from build123d import *

# Parameters (mm, degrees)
F1_DEPTH = 19.05
F2_DEPTH = 19.05
F3_DEPTH = 25.4


with BuildPart() as f1:
    # F0 (on Top) → F1 (new body)
    with BuildSketch(Plane.XY):
        with BuildLine():
            ThreePointArc((10.16, 0), (-4.399409, 9.1581), (-6.35, -7.931147))
            ThreePointArc((-6.35, -7.931147), (0, -10.16), (6.35, -7.931147))
            ThreePointArc((6.35, -7.931147), (9.1581, -4.399409), (10.16, 0))
        make_face()
    extrude(amount=F1_DEPTH)

    # F0 (on Top) → F2 (join)
    with BuildSketch(Plane.XY):
        with BuildLine():
            Line((-6.35, -7.931147), (-6.35, -24.593444))
            ThreePointArc((-6.35, -24.593444), (0, -25.4), (6.35, -24.593444))
            Line((6.35, -24.593444), (6.35, -7.931147))
            ThreePointArc((6.35, -7.931147), (0, -10.16), (-6.35, -7.931147))
        make_face()
    extrude(amount=F2_DEPTH)

    # F0 (on Top) → F3 (join)
    with BuildSketch(Plane.XY):
        with BuildLine():
            ThreePointArc((6.35, -24.593444), (20.080463, -15.55426), (25.4, 0))
            ThreePointArc((25.4, 0), (-15.55426, 20.080463), (-6.35, -24.593444))
            Line((-6.35, -24.593444), (-6.35, -7.931147))
            ThreePointArc((-6.35, -7.931147), (-4.399409, 9.1581), (10.16, 0))
            ThreePointArc((10.16, 0), (9.1581, -4.399409), (6.35, -7.931147))
            Line((6.35, -7.931147), (6.35, -24.593444))
        make_face()
    extrude(amount=F3_DEPTH)


solid = f1.part
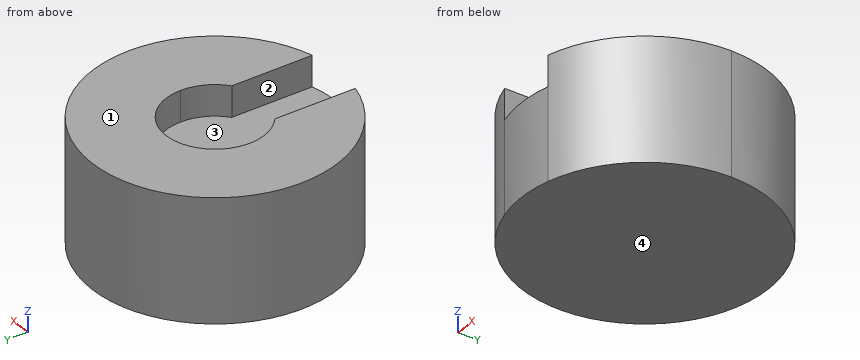
Work out the finished part from the listing and answer in its coordinate system (mm). Face numbers are marked on the shaded views. A direction names the side the tool comes from. Round coordinates to 2 decimals unless told otherwise and drop trailing zeros. Order: outer loops, then holes, each group sorted by start corner. A loop starts at its lowest first (then second) coordinate and runs counter-clockwise, first axis right, second up. Notation, with made-up numbers: M 3,62.5 L 29,62.5 A24 cw 29,83.5 Z; hole C 71,74.25 d6. An arc over 180 degrees is marked long. Put each result on its own line as item: value. Start each with the question number.
Q1. Section B-B, the plane y = -1.5 is taken. Write down the section's boundary in (x, z), and give its area (3 significant figures).
Q2. Straight lines are drawn through the part: L1, parallel to X at y = 0, z = 22.75; L2, parallel to Y at x = 0, z = 23.25; L3, parallel to X at y = 0.5, z = 16.5. For each, find the intervals that lie inside material, in ascending order. Write a range as [from, to].
Q3. Section D-D, the plane y = 8.5 is taken. Write down the section's boundary in (x, z), and give its area (3 significant figures).
Q4. Section C-C, the plane z = 7.75 is taken. Write down the section's boundary in (x, y), and give its area (3 significant figures).
Q5. A tool of negligible diameter and unlimited length cuts with its end or side. For the marked faces 3 and 4, from which of +Z, -Z, +X, -X, +Y, -Y can it reach the whole face along a straight path? Write none if from no direction.
Q6. Section A-A, the plane x = 0 is taken. Write down the section's boundary in (y, z), and give its area (3 significant figures).
Q7. Flat-ended cylindrical pins translate along their axes: pin 1 (10 mm diameter, centred on y = 11, z = 6.5, fed in from -X); pin 2 (4 mm diameter, centred on y = 5, z = 21.5, fed in from +X); pin 3 (5 mm diameter, centred on x = -16, z = 5.5, fed in from -Y). Find the tip coordinate at first contact, or state that the pin passes through.
Q8. For a pull along X with two mould halves and no side action, classify the marked faces 1 and 2 as pulls with the +X half, pulls with the -X half, needs draft (parallel to the pull), parting line crosses it, or undercut.
Findings below:
1. outline: M -25.36,0 L 25.36,0 L 25.36,25.4 L 10.05,25.4 L 10.05,19.05 L -10.05,19.05 L -10.05,25.4 L -25.36,25.4 Z
1. area: 1,160 mm^2
2. L1: x = [-25.4, -10.16], [10.16, 25.4]
2. L2: y = [10.16, 25.4]
2. L3: x = [-25.4, 25.4]
3. outline: M -23.94,0 L 23.94,0 L 23.94,25.4 L 5.57,25.4 L 5.57,19.05 L -5.57,19.05 L -5.57,25.4 L -23.94,25.4 Z
3. area: 1,150 mm^2
4. outline: M -6.35,-24.59 A25.4 ccw 6.35,-24.59 A25.4 ccw long Z
4. area: 2,030 mm^2
5. face 3: +Z
5. face 4: -Z, +X, -X, +Y, -Y
6. outline: M -25.4,0 L 25.4,0 L 25.4,25.4 L 10.16,25.4 L 10.16,19.05 L -25.4,19.05 Z
6. area: 1,060 mm^2
7. pin 1: stops at x = -24.68
7. pin 2: stops at x = 25.22
7. pin 3: stops at y = -21.52
8. face 1: needs draft
8. face 2: undercut
